Verification items for this drawing (mm, ordinates from the low corner). A direction names the side the tool comes from. Give positions to 0.01 mm unless a question says otherwise; leave off trailing zeros. Loops run counter-clockwise (first coordinate to the right, second up) from the corner with the lowest first, then second, coordinate; pieces in that order, holes last. Notation, with made-up numbers: (78, 0.5) - (123, 0.5) arc R25 ccw to (123, 39.5) - close; hole circle Ø6 at (41.5, -19). An arc over 180 degrees is marked (long way). One line per question, with ' | ' between items. Start each with the question number.
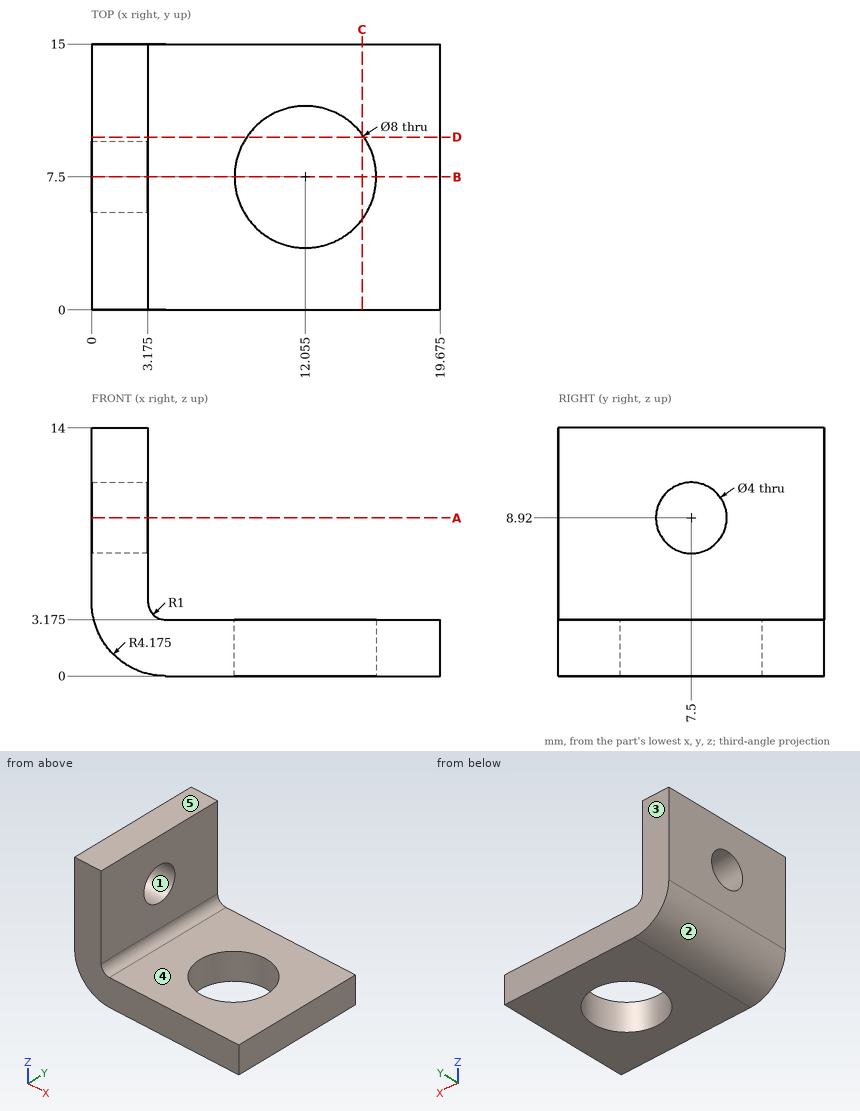
(1) Mould release check, pull along Y, two halves, no side actions. Record for the marked faces 1, 2 and 3: pulls with the +Y half, pulls with the -Y half, needs draft (parallel to the pull), parting line crosses it, or undercut.
(2) Section check C-C, the plane x = 15.25. Record the boundary of the cut face in (y, z) (3 decimals).
(3) Section check D-D, the plane y = 9.75. Record the boundary of the cut face in (x, z) (3 decimals), and give its area (3 significant figures).
(4) Depth check by flat-ended pin: pin 1 Ø3 at (y, z) = (8.5, 12) entering from +X (3 decimals); pin 2 Ø7.5 at (x, y) = (11, 7) entering from +Z (3 decimals); pin 3 Ø2 at (x, y) = (12.5, 6.5) entering from +Z; pin 4 Ø1 at (y, z) = (6.5, 3) entering from -X. Enter the tip coordinate at first touch or a pass-through.
(5) Section check B-B, the plane y = 7.5. Record the boundary of the cut face in (x, z) (3 decimals), and give its area (3 significant figures).
(6) Material ranges on line 1 (Y direction, x = 1.45, z = 8.92); line 2 (X direction, y = 0.75, z = 5.25) (3 decimals), recorded low to high.
(7) Tool access check on the marked faces 4 and 5. Record the directions out of +Z, -Z, +X, -X, +Y, -Y that give a thin tool (end or side, any length) a straight path to the whole face; none if there is none.
(8) Section check A-A, the plane z = 8.92. Record the boundary of the cut face in (x, y) (3 decimals).
Numbers:
1) face 1: undercut | face 2: needs draft | face 3: pulls with the +Y half
2) outline: (0, 0) - (5.093, 0) - (5.093, 3.175) - (0, 3.175) - close; (9.907, 0) - (15, 0) - (15, 3.175) - (9.907, 3.175) - close
3) outline: (0, 4.175) arc R4.175 ccw to (4.175, 0) - (8.748, 0) - (8.748, 3.175) - (4.175, 3.175) arc R1 cw to (3.175, 4.175) - (3.175, 14) - (0, 14) - close; (15.362, 0) - (19.675, 0) - (19.675, 3.175) - (15.362, 3.175) - close | area: 72.3 mm^2
4) pin 1: x = 3.175 | pin 2: z = 3.175 | pin 3: through | pin 4: x = 0.05
5) outline: (0, 4.175) arc R4.175 ccw to (4.175, 0) - (8.055, 0) - (8.055, 3.175) - (4.175, 3.175) arc R1 cw to (3.175, 4.175) - (3.175, 6.92) - (0, 6.92) - close; (0, 10.92) - (3.175, 10.92) - (3.175, 14) - (0, 14) - close; (16.055, 0) - (19.675, 0) - (19.675, 3.175) - (16.055, 3.175) - close | area: 55.2 mm^2
6) line 1: 0 to 5.5, 9.5 to 15 | line 2: 0 to 3.175
7) face 4: +Z, +X, +Y, -Y | face 5: +Z, +X, -X, +Y, -Y
8) outline: (0, 0) - (3.175, 0) - (3.175, 5.5) - (0, 5.5) - close; (0, 9.5) - (3.175, 9.5) - (3.175, 15) - (0, 15) - close
